from build123d import *

# Parameters (mm, degrees)
CROQUIS1_W               = 2.54
CROQUIS1_H               = 20.34
SALIENTE_EXTRUIR1_DEPTH  = 2.3
CORTAR_EXTRUIR4_DEPTH    = 2.3
CORTAR_EXTRUIR5_DEPTH    = 2.3
CORTAR_EXTRUIR6_DEPTH    = 2.3
CORTAR_EXTRUIR7_DEPTH    = 2.3
CORTAR_EXTRUIR8_DEPTH    = 2.3
CORTAR_EXTRUIR9_DEPTH    = 2.3
CORTAR_EXTRUIR10_DEPTH   = 2.3
CORTAR_EXTRUIR11_DEPTH   = 2.3
CORTAR_EXTRUIR12_DEPTH   = 2.3
CORTAR_EXTRUIR13_DEPTH   = 2.3
CORTAR_EXTRUIR14_DEPTH   = 2.3
CORTAR_EXTRUIR15_DEPTH   = 2.3
CORTAR_EXTRUIR16_DEPTH   = 2.3
CORTAR_EXTRUIR17_DEPTH   = 2.3
CORTAR_EXTRUIR18_DEPTH   = 2.3
CORTAR_EXTRUIR19_DEPTH   = 2.3
CROQUIS24_W              = 0.75
CROQUIS24_H              = 0.75
SALIENTE_EXTRUIR2_DEPTH  = 3.25
CROQUIS25_W              = 0.75
CROQUIS25_H              = 0.75
SALIENTE_EXTRUIR3_DEPTH  = 6.2
CROQUIS26_W              = 0.75
CROQUIS26_H              = 0.75
SALIENTE_EXTRUIR4_DEPTH  = 6.2
CROQUIS27_W              = 0.75
CROQUIS27_H              = 0.75
SALIENTE_EXTRUIR5_DEPTH  = 6.2
CROQUIS28_W              = 0.75
CROQUIS28_H              = 0.75
SALIENTE_EXTRUIR6_DEPTH  = 6.2
CROQUIS29_W              = 0.75
CROQUIS29_H              = 0.75
SALIENTE_EXTRUIR7_DEPTH  = 6.2
CROQUIS30_W              = 0.75
CROQUIS30_H              = 0.75
SALIENTE_EXTRUIR8_DEPTH  = 6.2
CROQUIS31_W              = 0.75
CROQUIS31_H              = 0.75
SALIENTE_EXTRUIR9_DEPTH  = 6.2
CROQUIS32_W              = 0.75
CROQUIS32_H              = 0.75
SALIENTE_EXTRUIR10_DEPTH = 6.2
CROQUIS37_W              = 0.75
CROQUIS37_H              = 0.75
SALIENTE_EXTRUIR15_DEPTH = 3.25
CROQUIS38_W              = 0.75
CROQUIS38_H              = 0.75
SALIENTE_EXTRUIR16_DEPTH = 3.25
CROQUIS39_W              = 0.75
CROQUIS39_H              = 0.75
SALIENTE_EXTRUIR17_DEPTH = 3.25
CROQUIS40_W              = 0.75
CROQUIS40_H              = 0.75
SALIENTE_EXTRUIR18_DEPTH = 3.25
CROQUIS41_W              = 0.75
CROQUIS41_H              = 0.75
SALIENTE_EXTRUIR19_DEPTH = 3.25
CROQUIS42_W              = 0.75
CROQUIS42_H              = 0.75
SALIENTE_EXTRUIR20_DEPTH = 3.25
CROQUIS43_W              = 0.75
CROQUIS43_H              = 0.75
SALIENTE_EXTRUIR21_DEPTH = 3.25
REDONDEO2_R              = 0.5


with BuildPart() as part:
    # Croquis1 → Saliente-Extruir1 (new body)
    with BuildSketch(Plane(origin=(0, 2.3, 0), x_dir=(1, 0, 0), z_dir=(0, 1, 0))):
        with Locations((0, -8.9)):
            Rectangle(CROQUIS1_W, CROQUIS1_H)
    extrude(amount=-SALIENTE_EXTRUIR1_DEPTH)

    # Croquis5 → Cortar-Extruir4 (cut)
    with BuildSketch(Plane.XZ):
        with BuildLine():
            Line((1.27, 18.55), (1.27, 19.55))
            ThreePointArc((1.27, 19.55), (1.123553391, 19.196446609), (0.77, 19.05))
            ThreePointArc((0.77, 19.05), (1.123553391, 18.903553391), (1.27, 18.55))
        make_face()
    extrude(amount=-CORTAR_EXTRUIR4_DEPTH, mode=Mode.SUBTRACT)

    # Croquis6 → Cortar-Extruir5 (cut)
    with BuildSketch(Plane.XZ):
        with BuildLine():
            Line((1.27, 16.01), (1.27, 17.01))
            ThreePointArc((1.27, 17.01), (1.123553391, 16.656446609), (0.77, 16.51))
            ThreePointArc((0.77, 16.51), (1.123553391, 16.363553391), (1.27, 16.01))
        make_face()
    extrude(amount=-CORTAR_EXTRUIR5_DEPTH, mode=Mode.SUBTRACT)

    # Croquis7 → Cortar-Extruir6 (cut)
    with BuildSketch(Plane.XZ):
        with BuildLine():
            Line((1.27, 13.47), (1.27, 14.47))
            ThreePointArc((1.27, 14.47), (1.123553391, 14.116446609), (0.77, 13.97))
            ThreePointArc((0.77, 13.97), (1.123553391, 13.823553391), (1.27, 13.47))
        make_face()
    extrude(amount=-CORTAR_EXTRUIR6_DEPTH, mode=Mode.SUBTRACT)

    # Croquis8 → Cortar-Extruir7 (cut)
    with BuildSketch(Plane.XZ):
        with BuildLine():
            Line((1.27, 10.93), (1.27, 11.93))
            ThreePointArc((1.27, 11.93), (1.123553391, 11.576446609), (0.77, 11.43))
            ThreePointArc((0.77, 11.43), (1.123553391, 11.283553391), (1.27, 10.93))
        make_face()
    extrude(amount=-CORTAR_EXTRUIR7_DEPTH, mode=Mode.SUBTRACT)

    # Croquis9 → Cortar-Extruir8 (cut)
    with BuildSketch(Plane.XZ):
        with BuildLine():
            Line((1.27, 8.39), (1.27, 9.39))
            ThreePointArc((1.27, 9.39), (1.123553391, 9.036446609), (0.77, 8.89))
            ThreePointArc((0.77, 8.89), (1.123553391, 8.743553391), (1.27, 8.39))
        make_face()
    extrude(amount=-CORTAR_EXTRUIR8_DEPTH, mode=Mode.SUBTRACT)

    # Croquis10 → Cortar-Extruir9 (cut)
    with BuildSketch(Plane.XZ):
        with BuildLine():
            Line((1.27, 5.85), (1.27, 6.85))
            ThreePointArc((1.27, 6.85), (1.123553391, 6.496446609), (0.77, 6.35))
            ThreePointArc((0.77, 6.35), (1.123553391, 6.203553391), (1.27, 5.85))
        make_face()
    extrude(amount=-CORTAR_EXTRUIR9_DEPTH, mode=Mode.SUBTRACT)

    # Croquis11 → Cortar-Extruir10 (cut)
    with BuildSketch(Plane.XZ):
        with BuildLine():
            Line((1.27, 3.31), (1.27, 4.31))
            ThreePointArc((1.27, 4.31), (1.123553391, 3.956446609), (0.77, 3.81))
            ThreePointArc((0.77, 3.81), (1.123553391, 3.663553391), (1.27, 3.31))
        make_face()
    extrude(amount=-CORTAR_EXTRUIR10_DEPTH, mode=Mode.SUBTRACT)

    # Croquis12 → Cortar-Extruir11 (cut)
    with BuildSketch(Plane.XZ):
        with BuildLine():
            Line((1.27, 0.77), (1.27, 1.77))
            ThreePointArc((1.27, 1.77), (1.123553391, 1.416446609), (0.77, 1.27))
            ThreePointArc((0.77, 1.27), (1.123553391, 1.123553391), (1.27, 0.77))
        make_face()
    extrude(amount=-CORTAR_EXTRUIR11_DEPTH, mode=Mode.SUBTRACT)

    # Croquis13 → Cortar-Extruir12 (cut)
    with BuildSketch(Plane.XZ):
        with BuildLine():
            Line((-1.27, 1.77), (-1.27, 0.77))
            ThreePointArc((-1.27, 0.77), (-1.123553391, 1.123553391), (-0.77, 1.27))
            ThreePointArc((-0.77, 1.27), (-1.123553391, 1.416446609), (-1.27, 1.77))
        make_face()
    extrude(amount=-CORTAR_EXTRUIR12_DEPTH, mode=Mode.SUBTRACT)

    # Croquis14 → Cortar-Extruir13 (cut)
    with BuildSketch(Plane.XZ):
        with BuildLine():
            Line((-1.27, 4.31), (-1.27, 3.31))
            ThreePointArc((-1.27, 3.31), (-1.123553391, 3.663553391), (-0.77, 3.81))
            ThreePointArc((-0.77, 3.81), (-1.123553391, 3.956446609), (-1.27, 4.31))
        make_face()
    extrude(amount=-CORTAR_EXTRUIR13_DEPTH, mode=Mode.SUBTRACT)

    # Croquis15 → Cortar-Extruir14 (cut)
    with BuildSketch(Plane.XZ):
        with BuildLine():
            Line((-1.27, 6.85), (-1.27, 5.85))
            ThreePointArc((-1.27, 5.85), (-1.123553391, 6.203553391), (-0.77, 6.35))
            ThreePointArc((-0.77, 6.35), (-1.123553391, 6.496446609), (-1.27, 6.85))
        make_face()
    extrude(amount=-CORTAR_EXTRUIR14_DEPTH, mode=Mode.SUBTRACT)

    # Croquis16 → Cortar-Extruir15 (cut)
    with BuildSketch(Plane.XZ):
        with BuildLine():
            Line((-1.27, 9.39), (-1.27, 8.39))
            ThreePointArc((-1.27, 8.39), (-1.123553391, 8.743553391), (-0.77, 8.89))
            ThreePointArc((-0.77, 8.89), (-1.123553391, 9.036446609), (-1.27, 9.39))
        make_face()
    extrude(amount=-CORTAR_EXTRUIR15_DEPTH, mode=Mode.SUBTRACT)

    # Croquis17 → Cortar-Extruir16 (cut)
    with BuildSketch(Plane.XZ):
        with BuildLine():
            Line((-1.27, 11.93), (-1.27, 10.93))
            ThreePointArc((-1.27, 10.93), (-1.123553391, 11.283553391), (-0.77, 11.43))
            ThreePointArc((-0.77, 11.43), (-1.123553391, 11.576446609), (-1.27, 11.93))
        make_face()
    extrude(amount=-CORTAR_EXTRUIR16_DEPTH, mode=Mode.SUBTRACT)

    # Croquis18 → Cortar-Extruir17 (cut)
    with BuildSketch(Plane.XZ):
        with BuildLine():
            Line((-1.27, 14.47), (-1.27, 13.47))
            ThreePointArc((-1.27, 13.47), (-1.123553391, 13.823553391), (-0.77, 13.97))
            ThreePointArc((-0.77, 13.97), (-1.123553391, 14.116446609), (-1.27, 14.47))
        make_face()
    extrude(amount=-CORTAR_EXTRUIR17_DEPTH, mode=Mode.SUBTRACT)

    # Croquis19 → Cortar-Extruir18 (cut)
    with BuildSketch(Plane.XZ):
        with BuildLine():
            Line((-1.27, 17.01), (-1.27, 16.01))
            ThreePointArc((-1.27, 16.01), (-1.123553391, 16.363553391), (-0.77, 16.51))
            ThreePointArc((-0.77, 16.51), (-1.123553391, 16.656446609), (-1.27, 17.01))
        make_face()
    extrude(amount=-CORTAR_EXTRUIR18_DEPTH, mode=Mode.SUBTRACT)

    # Croquis20 → Cortar-Extruir19 (cut)
    with BuildSketch(Plane.XZ):
        with BuildLine():
            Line((-1.27, 19.55), (-1.27, 18.55))
            ThreePointArc((-1.27, 18.55), (-1.123553391, 18.903553391), (-0.77, 19.05))
            ThreePointArc((-0.77, 19.05), (-1.123553391, 19.196446609), (-1.27, 19.55))
        make_face()
    extrude(amount=-CORTAR_EXTRUIR19_DEPTH, mode=Mode.SUBTRACT)

    # Croquis24 → Saliente-Extruir2 (add)
    with BuildSketch(Plane.XZ):
        Rectangle(CROQUIS24_W, CROQUIS24_H)
    extrude(amount=SALIENTE_EXTRUIR2_DEPTH)

    # Croquis25 → Saliente-Extruir3 (add)
    with BuildSketch(Plane(origin=(0, 2.3, 0), x_dir=(-1, 0, 0), z_dir=(0, 1, 0))):
        Rectangle(CROQUIS25_W, CROQUIS25_H)
    extrude(amount=SALIENTE_EXTRUIR3_DEPTH)

    # Croquis26 → Saliente-Extruir4 (add)
    with BuildSketch(Plane(origin=(0, 2.3, 0), x_dir=(-1, 0, 0), z_dir=(0, 1, 0))):
        with Locations((0, 2.54)):
            Rectangle(CROQUIS26_W, CROQUIS26_H)
    extrude(amount=SALIENTE_EXTRUIR4_DEPTH)

    # Croquis27 → Saliente-Extruir5 (add)
    with BuildSketch(Plane(origin=(0, 2.3, 0), x_dir=(-1, 0, 0), z_dir=(0, 1, 0))):
        with Locations((0, 5.08)):
            Rectangle(CROQUIS27_W, CROQUIS27_H)
    extrude(amount=SALIENTE_EXTRUIR5_DEPTH)

    # Croquis28 → Saliente-Extruir6 (add)
    with BuildSketch(Plane(origin=(0, 2.3, 0), x_dir=(-1, 0, 0), z_dir=(0, 1, 0))):
        with Locations((0, 7.62)):
            Rectangle(CROQUIS28_W, CROQUIS28_H)
    extrude(amount=SALIENTE_EXTRUIR6_DEPTH)

    # Croquis29 → Saliente-Extruir7 (add)
    with BuildSketch(Plane(origin=(0, 2.3, 0), x_dir=(-1, 0, 0), z_dir=(0, 1, 0))):
        with Locations((0, 10.16)):
            Rectangle(CROQUIS29_W, CROQUIS29_H)
    extrude(amount=SALIENTE_EXTRUIR7_DEPTH)

    # Croquis30 → Saliente-Extruir8 (add)
    with BuildSketch(Plane(origin=(0, 2.3, 0), x_dir=(-1, 0, 0), z_dir=(0, 1, 0))):
        with Locations((0, 12.7)):
            Rectangle(CROQUIS30_W, CROQUIS30_H)
    extrude(amount=SALIENTE_EXTRUIR8_DEPTH)

    # Croquis31 → Saliente-Extruir9 (add)
    with BuildSketch(Plane(origin=(0, 2.3, 0), x_dir=(-1, 0, 0), z_dir=(0, 1, 0))):
        with Locations((0, 15.24)):
            Rectangle(CROQUIS31_W, CROQUIS31_H)
    extrude(amount=SALIENTE_EXTRUIR9_DEPTH)

    # Croquis32 → Saliente-Extruir10 (add)
    with BuildSketch(Plane(origin=(0, 2.3, 0), x_dir=(-1, 0, 0), z_dir=(0, 1, 0))):
        with Locations((0, 17.78)):
            Rectangle(CROQUIS32_W, CROQUIS32_H)
    extrude(amount=SALIENTE_EXTRUIR10_DEPTH)

    # Croquis37 → Saliente-Extruir15 (add)
    with BuildSketch(Plane.XZ):
        with Locations((0, 2.54)):
            Rectangle(CROQUIS37_W, CROQUIS37_H)
    extrude(amount=SALIENTE_EXTRUIR15_DEPTH)

    # Croquis38 → Saliente-Extruir16 (add)
    with BuildSketch(Plane.XZ):
        with Locations((0, 5.08)):
            Rectangle(CROQUIS38_W, CROQUIS38_H)
    extrude(amount=SALIENTE_EXTRUIR16_DEPTH)

    # Croquis39 → Saliente-Extruir17 (add)
    with BuildSketch(Plane.XZ):
        with Locations((0, 7.62)):
            Rectangle(CROQUIS39_W, CROQUIS39_H)
    extrude(amount=SALIENTE_EXTRUIR17_DEPTH)

    # Croquis40 → Saliente-Extruir18 (add)
    with BuildSketch(Plane.XZ):
        with Locations((0, 10.16)):
            Rectangle(CROQUIS40_W, CROQUIS40_H)
    extrude(amount=SALIENTE_EXTRUIR18_DEPTH)

    # Croquis41 → Saliente-Extruir19 (add)
    with BuildSketch(Plane.XZ):
        with Locations((0, 12.7)):
            Rectangle(CROQUIS41_W, CROQUIS41_H)
    extrude(amount=SALIENTE_EXTRUIR19_DEPTH)

    # Croquis42 → Saliente-Extruir20 (add)
    with BuildSketch(Plane.XZ):
        with Locations((0, 15.24)):
            Rectangle(CROQUIS42_W, CROQUIS42_H)
    extrude(amount=SALIENTE_EXTRUIR20_DEPTH)

    # Croquis43 → Saliente-Extruir21 (add)
    with BuildSketch(Plane.XZ):
        with Locations((0, 17.78)):
            Rectangle(CROQUIS43_W, CROQUIS43_H)
    extrude(amount=SALIENTE_EXTRUIR21_DEPTH)

    # Redondeo2
    redondeo2_edges = [part.edges().sort_by_distance(p)[0] for p in [
        (-1.27, 1.15, -1.27),
        (1.27, 1.15, -1.27),
    ]]
    fillet(redondeo2_edges, radius=REDONDEO2_R)


solid = part.part
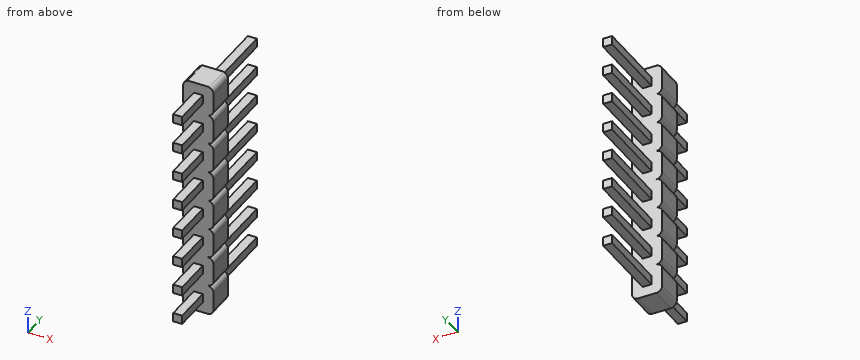
Here's how the part is built. I have some questions about the finished solid (model axes, mm). Coordinates: 2 decimals unless noted, no trailing zeros. Write each loop counter-clockwise with the first axis right and the second up, starting at its lowest first coordinate (ties: lowest second). Pieces come first, ordered by that corner, then holes.
1) I'm going to push flat-ended pins straight in: pin 1 (0.6 mm diameter, centred on y = -2, z = 10, fed in from +X) (3 decimals); pin 2 (0.6 mm diameter, centred on y = 4.5, z = 12.5, fed in from -X) (3 decimals); pin 3 (0.6 mm diameter, centred on x = 0, y = 5.5, fed in from +Z) (3 decimals). Where does each tip first touch, or does it pass through?
Filled in:
pin 1: stops at x = 0.375
pin 2: stops at x = -0.375
pin 3: stops at z = 18.155
2) If we section it at A-A (y = 5.25): Count the separate pieces of the cut face and the enclosed holes in it, plus the area to 3 significant figures.
Filled in:
separate pieces: 8
enclosed holes: 0
area: 4.50 mm2
3) If I drill on line 1 (Y direction, x = 1.15, z = 2); line 2 (X direction, y = 4.5, z = 10.25) (3 decimals); line 3 (X direction, y = 1, z = 4), over which ranges is the centre line in solid material (lowest first)?
Filled in:
line 1: y = 0 to 2.3
line 2: x = -0.375 to 0.375
line 3: x = -1.16 to 1.16
4) If we section it at B-B (z = 2.5): List the corners of the cut face in (x, y) for me (3 decimals).
Filled in:
outline: (-1.27, 0) - (-0.375, 0) - (-0.375, -3.25) - (0.375, -3.25) - (0.375, 0) - (1.27, 0) - (1.27, 2.3) - (0.375, 2.3) - (0.375, 8.5) - (-0.375, 8.5) - (-0.375, 2.3) - (-1.27, 2.3) - close
